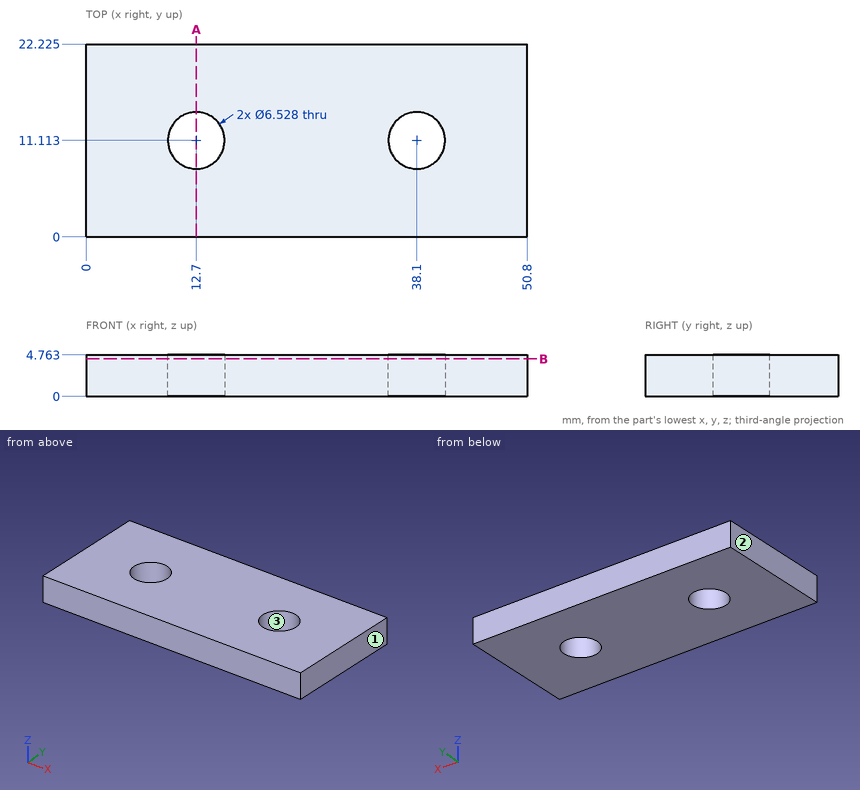
Design review of the part shown in the three views and the two pictorial views. Dimensions are in mm from the part's minimum x, y and z. Round coordinates to 2 decimals unless told otherwise and drop trailing zeros. Write each loop counter-clockwise with the first axis right and the second up, starting at its lowest first coordinate (ties: lowest second). Pieces come first, ordered by that corner, then holes. Notation, with made-up numbers: (-24.75, 14.5) -> (1.25, 14.5) arc R19 ccw to (1.25, 43.5) -> close; hole circle Ø4 at (6, 87.5). An arc over 180 degrees is marked (long way). Answer as a JSON object with one key per item and string values.
1. We need section B-B on z = 4.3. State the section outline as (x, y) points (1 decimal).
Results found:
{"outline": "(0, 0) -> (50.8, 0) -> (50.8, 22.2) -> (0, 22.2) -> close; hole circle Ø6.5 at (12.7, 11.1); hole circle Ø6.5 at (38.1, 11.1)"}
2. The part is to be moulded in two halves that separate along X. For the marked faces 1, 2 and 3, say which applies: pulls with the +X half, pulls with the -X half, needs draft (parallel to the pull), parting line crosses it, or undercut.
Results found:
{"face 1": "pulls with the +X half", "face 2": "pulls with the -X half", "face 3": "undercut"}
3. Clearance check with flat-ended pins moving along their axes: pin 1 (1 mm diameter, centred on x = 31, z = 0.5, fed in from -Y); pin 2 (6 mm diameter, centred on x = 12.7, y = 11.11, fed in from +Z). State where each tip first meets the part, or that it passes through.
Results found:
{"pin 1": "stops at y = 0", "pin 2": "passes through"}
4. To check wall thickness, follow line 1 along X through (y, z) = (11.75, 4.1); line 2 along X through (y, z) = (9.75, 1.55) (1 decimal); line 3 along Y through (x, z) = (12.7, 2.4) (1 decimal). State the ranges of each line that lie inside material, in increasing order.
Results found:
{"line 1": "x = 0 to 9.5, 15.9 to 34.9, 41.3 to 50.8", "line 2": "x = 0 to 9.7, 15.7 to 35.1, 41.1 to 50.8", "line 3": "y = 0 to 7.8, 14.4 to 22.2"}
5. We need section A-A on x = 12.7. State the section outline as (y, z) points (1 decimal).
Results found:
{"outline": "(0, 0) -> (7.8, 0) -> (7.8, 4.8) -> (0, 4.8) -> close; (14.4, 0) -> (22.2, 0) -> (22.2, 4.8) -> (14.4, 4.8) -> close"}
